The drawing under review shows one solid part. Ordinate dimensions are in mm from its lowest x, y, z. A direction names the side the tool comes from. Coordinates: 2 decimals unless noted, no trailing zeros. Loops run counter-clockwise (first coordinate to the right, second up) from the corner with the lowest first, then second, coordinate; pieces in that order, holes last. Notation, with made-up numbers: (5, 88.5) -> (62, 88.5) arc R20 ccw to (62, 103.5) -> close; hole circle Ø8 at (-31, 56). An arc over 180 degrees is marked (long way). Use a Markdown table: item, result.
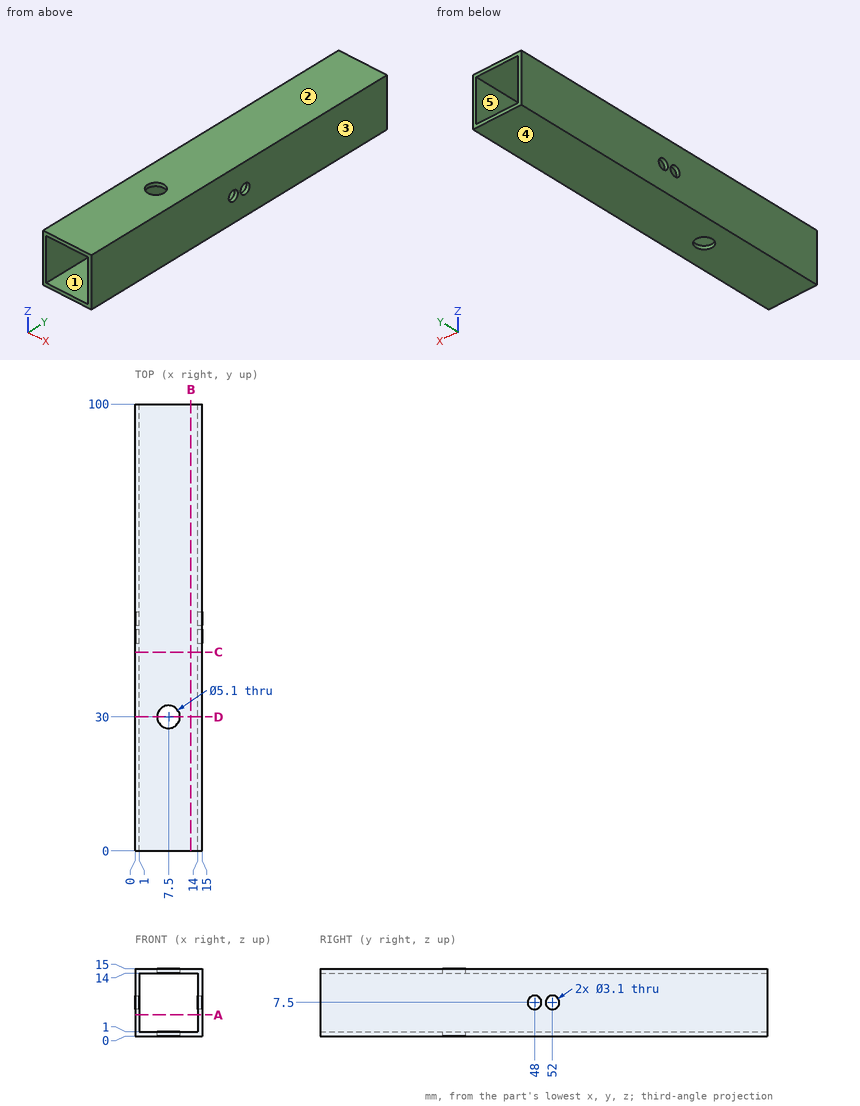
(1) Take a section at D-D on y = 30. Write out the cut boundary in (x, z).
Found:
| item | result |
|---|---|
| outline | (0, 0) -> (4.95, 0) -> (4.95, 1) -> (1, 1) -> (1, 14) -> (4.95, 14) -> (4.95, 15) -> (0, 15) -> close; (10.05, 0) -> (15, 0) -> (15, 15) -> (10.05, 15) -> (10.05, 14) -> (14, 14) -> (14, 1) -> (10.05, 1) -> close |
(2) Take a section at C-C on y = 44.5. Write out the cut boundary in (x, z).
Found:
| item | result |
|---|---|
| outline | (0, 0) -> (15, 0) -> (15, 15) -> (0, 15) -> close; hole (1, 1) -> (14, 1) -> (14, 14) -> (1, 14) -> close |
(3) For line 1 along Y through (x, z) = (14.55, 7.5); line 2 along Z through (x, y) = (11.5, 19), list the stretches that pass through material, from the lowest coordinate up.
Found:
| item | result |
|---|---|
| line 1 | y = 0 to 46.45, 49.55 to 50.45, 53.55 to 100 |
| line 2 | z = 0 to 1, 14 to 15 |
(4) For the marked faces 1 and 2, list the 3-axis set-ups (+Z, -Z, +X, -X, +Y, -Y) from which the entire face can be reached by the end or side of a thin tool; tool diameter is ignored.
Found:
| item | result |
|---|---|
| face 1 | +Y, -Y |
| face 2 | +Z, +X, -X, +Y, -Y |
(5) Take a section at A-A on z = 4.75. Write out the cut boundary in (x, y).
Found:
| item | result |
|---|---|
| outline | (0, 0) -> (1, 0) -> (1, 100) -> (0, 100) -> close; (14, 0) -> (15, 0) -> (15, 100) -> (14, 100) -> close |
(6) Take a section at B-B on x = 12.5. Write out the cut boundary in (y, z).
Found:
| item | result |
|---|---|
| outline | (0, 0) -> (100, 0) -> (100, 1) -> (0, 1) -> close; (0, 14) -> (100, 14) -> (100, 15) -> (0, 15) -> close |
(7) Mouldability with a two-part tool opening along X and no side actions: class the marked faces 3, 4 and 5 as pulls with the +X half, pulls with the -X half, needs draft (parallel to the pull), parting line crosses it, or undercut.
Found:
| item | result |
|---|---|
| face 3 | pulls with the +X half |
| face 4 | needs draft |
| face 5 | undercut |
(8) For pin 1 Ø6 at (x, y) = (7.5, 30) entering from -Z, flat-tipped, find the tip position at first contact; note if it passes through.
Found:
| item | result |
|---|---|
| pin 1 | stops at z = 0 |
